Source: CAD feature listing. Evaluate the final solid. Frame: model axes, mm. A direction names the side the tool comes from. Coordinates: 2 decimals unless noted, no trailing zeros. Order: outer loops, then holes, each group sorted by start corner. A loop starts at its lowest first (then second) coordinate and runs counter-clockwise, first axis right, second up.
```python
from build123d import *

# Parameters (mm, degrees)
CHAMFER_1_SIZE = 1


with BuildPart() as part:
    # 草图1 → 旋转1 (revolve)
    with BuildSketch(Plane.XY):
        Polygon((0, 0), (10, 0), (10, -25), (7.5, -25), (7.5, -45), (0, -45), align=None)
    revolve(axis=Axis((0, -45, 0), (0, 1, 0)))

    # 倒角1
    chamfer_1_edges = [part.edges().sort_by_distance(p)[0] for p in [
        (-7.5, -45, 0),
        (-10, 0, 0),
    ]]
    chamfer(chamfer_1_edges, length=CHAMFER_1_SIZE)


solid = part.part
```
1. Section query A-A on z = 0. Return loops of the section in (x, y), plus the area to 3 significant figures.
Findings:
outline: (-10, -25) - (-7.5, -25) - (-7.5, -44) - (-6.5, -45) - (6.5, -45) - (7.5, -44) - (7.5, -25) - (10, -25) - (10, -1) - (9, 0) - (-9, 0) - (-10, -1) - close
area: 798 mm2
2. Ray query, line 1 (X direction, y = -39, z = 0); line 2 (X direction, y = -5.5, z = 2.5); line 3 (Y direction, x = -6.75, z = 3.75). Return the intervals inside material, ascending.
Findings:
line 1: x = -7.5 to 7.5
line 2: x = -9.68 to 9.68
line 3: y = -25 to 0
3. Section query D-D on y = -36. Return loops of the section in (x, z).
Findings:
outline: circle Ø15 at (0, 0)
4. Access query for faces 1 (the face through (-7.493, -34.633, -0.33)), 2 (the face through (-2.17, -13.17, 9.76)). Directions: +Z, -Z, +X, -X, +Y, -Y. A direction counts if a zero-diameter tool reaches every point of the face in a straight line with its end or side. Return the directions, or none.
Findings:
face 1: -Y
face 2: +Y, -Y
5. Pin query (flat end, axial travel): P1, Ø6, axis at y = -37.5, z = 7, coming from the -X side; P2, Ø1.5, axis at x = -6, y = -6, coming from the +Z side; P3, Ø1, axis at x = 2, y = -5.5, coming from the +Z side. Return the tip coordinate at first contact, or that it passes through.
Findings:
P1: stops at x = -6.34
P2: stops at z = 8.51
P3: stops at z = 9.89
6. Section query B-B on x = 0. Return loops of the section in (y, z), plus the area to 3 significant figures.
Findings:
outline: (-45, -6.5) - (-44, -7.5) - (-25, -7.5) - (-25, -10) - (-1, -10) - (0, -9) - (0, 9) - (-1, 10) - (-25, 10) - (-25, 7.5) - (-44, 7.5) - (-45, 6.5) - close
area: 798 mm2
7. Section query C-C on y = -14. Return loops of the section in (x, z).
Findings:
outline: circle Ø20 at (0, 0)
